Read the model definition and answer for the solid it produces. Units are mm, in the model's axes. A direction names the side the tool comes from. Give positions to 0.01 mm unless a question says otherwise; leave off trailing zeros. Write each loop counter-clockwise with the first axis right and the second up, starting at its lowest first coordinate (ties: lowest second). Pieces come first, ordered by that corner, then holes. Notation, with made-up numbers: (-35.5, 32) -> (7.5, 32) arc R32 ccw to (7.5, 64) -> close; hole circle Ø5 at (-6.75, 47). An arc over 180 degrees is marked (long way). Put each result on its own line as item: value. Start each with the question number.
from build123d import *

# Parameters (mm, degrees)
SKETCH2_R                = 27
BOSS_EXTRUDE1_DEPTH      = 3.175
F_5_16_CLEARANCE_HOLE1_D = 8.4328
F_1_4_CLEARANCE_HOLE1_D  = 6.7564
CIRPATTERN1_COUNT        = 6


with BuildPart() as part:
    # Sketch2 → Boss-Extrude1 (new body, symmetric)
    with BuildSketch(Plane.XY):
        Circle(SKETCH2_R)
    extrude(amount=BOSS_EXTRUDE1_DEPTH, both=True)

    # 5/16 Clearance Hole1 (through all)
    with Locations(Plane.XY.offset(3.175)):
        with Locations((0, 0)):
            Hole(F_5_16_CLEARANCE_HOLE1_D / 2)

    # 1/4 Clearance Hole1 (through all)
    with Locations(Plane.XY.offset(3.175)):
        with Locations((-15.875, 0), (15.875, 0)):
            Hole(F_1_4_CLEARANCE_HOLE1_D / 2)

    # Sketch9 → Tap Drill for #6-32 Tap1 (revolve, cut)
    with BuildSketch(Plane(origin=(0, 27, 0), x_dir=(0, 0, 1), z_dir=(1, 0, 0))):
        Polygon((0, 0), (0, 7.16269403), (1.35255, 6.35), (1.35255, 0), align=None)
    tap_drill_for_6_32_tap1 = revolve(axis=Axis((0, 33.35, 0), (0, -1, 0)), mode=Mode.SUBTRACT)

    # CirPattern1: Tap Drill for #6-32 Tap1 ×6 about axis
    cirpattern1_axis = Axis((0, 0, 3.175), (0, 0, 1))
    for i in range(1, CIRPATTERN1_COUNT):
        add(tap_drill_for_6_32_tap1.rotate(cirpattern1_axis, i * 360 / CIRPATTERN1_COUNT), mode=Mode.SUBTRACT)


solid = part.part
1) A cutting plane is placed at D-D on y = 6.5. Give the vertices of the cut face in (x, z) (3 decimals).
2) A cutting plane is placed at B-B on z = -2. Give the vertices of the cut face in (x, y) (3 decimals).
3) A cutting plane is placed at C-C on x = -8.5. Give the vertices of the cut face in (y, z) (3 decimals).
4) For faces 1 (the face through (17.203, 10.161, 0.126)), 2 (the face through (-1.32, -23.87, -0.29)), 3 (the face through (-1.14, 23.87, 0.73)), 4 (the face through (6, 0, -3.175)), determine the directions among +Z, -Z, +X, -X, +Y, -Y from which every point of the face is accessible in a straight line to the end or side of a thin tool.
5) For a pull along Z with two mould halves and no side action, classify faces 5 (the face through (-18.996, -1.294, -0.044)), 6 (the face through (6, 0, 3.175)), 7 (the face through (-17.406, -9.809, 0.108)) as pulls with the +Z half, pulls with the -Z half, needs draft (parallel to the pull), parting line crosses it, or undercut.
6) A cutting plane is placed at A-A on y = 0. Give the vertices of the cut face in (x, z) (3 decimals).
7) Each of these flat-tipped pins is pushed along its axis until it touches: pin 1 Ø3 at (x, z) = (11, -1) entering from +Y; pin 2 Ø5.5 at (x, y) = (-15.875, 0) entering from -Z; pin 3 Ø3 at (x, z) = (0, 0) entering from -Y; pin 4 Ø1 at (x, z) = (14.5, -1) entering from +Y. Where does it stop, or does it pass through?
8) Straight lines are drawn through the part: line 1 (Z direction, x = 0, y = -25.5) (3 decimals); line 2 (Y direction, x = 0, z = 0); line 3 (Y direction, x = -20, z = 1). For each, find the intervals that lie inside material, in ascending order. Write a range as [from, to].
Results found:
1. outline: (-26.206, -3.175) -> (26.206, -3.175) -> (26.206, 3.175) -> (-26.206, 3.175) -> close
2. outline: circle Ø54 at (0, 0); hole circle Ø6.756 at (-15.875, 0); hole circle Ø8.433 at (0, 0); hole circle Ø6.756 at (15.875, 0)
3. outline: (-25.627, -3.175) -> (25.627, -3.175) -> (25.627, 3.175) -> (-25.627, 3.175) -> close
4. face 1: none
4. face 2: -Y
4. face 3: +Y
4. face 4: -Z, +X, -X, +Y, -Y
5. face 5: needs draft
5. face 6: pulls with the +Z half
5. face 7: undercut
6. outline: (-27, -3.175) -> (-19.253, -3.175) -> (-19.253, 3.175) -> (-27, 3.175) -> close; (-12.497, -3.175) -> (-4.216, -3.175) -> (-4.216, 3.175) -> (-12.497, 3.175) -> close; (4.216, -3.175) -> (12.497, -3.175) -> (12.497, 3.175) -> (4.216, 3.175) -> close; (19.253, -3.175) -> (27, -3.175) -> (27, 3.175) -> (19.253, 3.175) -> close
7. pin 1: stops at y = 25.27
7. pin 2: passes through
7. pin 3: stops at y = -27
7. pin 4: stops at y = 23.09
8. line 1: z = [-3.175, -1.353], [1.353, 3.175]
8. line 2: y = [-19.84, -4.22], [4.22, 19.84]
8. line 3: y = [-18.14, -12.6], [-10.5, 10.5], [12.6, 18.14]
